Autodesk Inventor part; units mm, degrees
ref_plane "Work Plane2" through (-109.0183, 0, 0) normal (-1, 0, 0) x (0, 0, 1)
ref_plane "Work Plane3" through (200, 0, 0) normal (-0.9782514, 0.2074228, 0) x (0, 0, 1)
ref_plane "Section Plane" through (-106.6132, -40.9526, 0) normal (0.99828, 0.058627, 0) x (0, 0, 1)
ref_plane "Work Plane2" through (-109.0183, 0, 0) normal (-1, 0, 0) x (0, 0, 1)
ref_plane "Work Plane3" through (200, 0, 0) normal (-0.9782514, 0.2074228, 0) x (0, 0, 1)
sketch "Path" plane through (0, 0, 0) normal (0, 0, 1) x (1, 0, 0)
  arc A0 (-106.6132, 40.9526) -> (-106.6132, -40.9526) centre (-109.0183, 0) ccw
  arc A1 (201.3429, -22.867) -> (201.3429, 22.867) centre (200, 0) ccw
  line L0 (201.3429, -22.867) -> (-106.6132, -40.9526)
  line L1 (-106.6132, 40.9526) -> (201.3429, 22.867)
  dimension "d31" = 8.26
ref_plane "Section Plane" through (-106.6132, -40.9526, 0) normal (0.99828, 0.058627, 0) x (0, 0, 1)
sketch "Section Sketch" plane through (-106.6132, -40.9526, 0) normal (0.99828, 0.058627, 0) x (0, 0, 1)
  line L0 (-6.75, -1.64) -> (6.75, -1.64)
  line L1 (6.75, -1.64) -> (6.75, 1.64)
  line L2 (6.75, 1.64) -> (-6.75, 1.64)
  line L3 (-6.75, 1.64) -> (-6.75, -1.64)
  line L4 (-2.86, -3.175) -> (2.86, -3.175)
  line L5 (2.86, -3.175) -> (2.86, 3.175)
  line L6 (2.86, 3.175) -> (-2.86, 3.175)
  line L7 (-2.86, 3.175) -> (-2.86, -3.175)
  line L8 (-2.86, 0) -> (2.86, 0) construction
  line L9 (-5.16, -4.13) -> (-2.86, -4.13)
  line L10 (-2.86, -4.13) -> (-2.86, 4.13)
  line L11 (-2.86, 4.13) -> (-5.16, 4.13)
  line L12 (-5.16, 4.13) -> (-5.16, -4.13)
  line L13 (2.86, -4.13) -> (5.16, -4.13)
  line L14 (5.16, -4.13) -> (5.16, 4.13)
  line L15 (5.16, 4.13) -> (2.86, 4.13)
  line L16 (2.86, 4.13) -> (2.86, -4.13)
  line L17 (-6.75, 0) -> (6.75, 0) construction
  point P0 (0, 0)
  point P1 (0, 0)
  dimension "d21" = 3.28
  dimension "d22" = 6.35
  dimension "d23" = 5.72
  dimension "d24" = 2.3
  dimension "d31" = 8.26
  dimension "d32" = 13.5
sweep "Solid" add profiles "Section Sketch" path "Path"
pattern_of_one "Strand Pattern"
equation "\"d21\" = da_d2"
equation "\"d22\" = da_d1"
equation "\"d23\" = da_b1"
equation "\"d24\" = da_t1 + da_t2"
equation "\"d30\" = da_pt"
equation "\"da_p\" = 9.525"
equation "\"da_b1\" = 5.72"
equation "\"da_h2\" = 8.26"
equation "\"da_h3\" = 8.26"
equation "\"da_d1\" = 6.35"
equation "\"da_d2\" = 3.28"
equation "\"da_pt\" = 10.24"
equation "\"da_b\" = 13.5"
equation "\"da_t1\" = 1.3"
equation "\"da_t2\" = 1"
properties part number "Roller Chain"
The model under review builds one solid part; all positions refer to its coordinate system, in mm. A direction names the side the tool comes from. Coordinates: 2 decimals unless noted, no trailing zeros. Answer as a JSON object with one key per item and string values. Group by question number.
1. To check wall thickness, follow probe 1 along Z at (x, y) = (54, 28); probe 2 along Y at (x, z) = (-124, 0.5); probe 3 along Y at (x, z) = (84, 4). State the ranges of each line that lie inside material, in increasing order.
2. Mouldability with a two-part tool opening along X and no side actions: class faces 4 (the face through (39, -29, 5.16)), 5 (the face through (45.45, 36.16, -3.99)), 6 (the face through (45.1, 30.4, 5.9)) as pulls with the +X half, pulls with the -X half, needs draft (parallel to the pull), parting line crosses it, or undercut.
3. Machinability: for faces 1 (the face through (-146.857, 0.863, 0.04)), 2 (the face through (-145.9, 0.84, 4.03)), 3 (the face through (-148.39, 0.9, -5.94)), which of the approach directions +Z, -Z, +X, -X, +Y, -Y give a long, thin tool a straight path to every point of the face, cutting with its end or side? Answer none if there is none.
4. Clearance check with flat-ended pins moving along their axes: pin 1 Ø6 at (x, z) = (107, -2.5) entering from +Y; pin 2 Ø2 at (x, y) = (-20, -29) entering from -Z; pin 3 Ø3 at (y, z) = (7.5, -3.5) entering from -X; pin 4 Ø4 at (y, z) = (19, -2.5) entering from +X. State where each tip first meets the part, or that it passes through.
Findings:
{
 "1": {"probe 1": "-5.16 to -2.86, 2.86 to 5.16", "probe 2": "-41.58 to -34.76, 34.76 to 41.58", "probe 3": "-33.9 to -25.62, 25.62 to 33.9"},
 "2": {"face 4": "undercut", "face 5": "pulls with the +X half", "face 6": "undercut"},
 "3": {"face 1": "none", "face 2": "+Z, -Z", "face 3": "-Z"},
 "4": {"pin 1": "y = 32.72", "pin 2": "through", "pin 3": "x = -153.77", "pin 4": "x = 221"}
}
